Part print with two shaded views. Sizes in mm from the minimum x, y, z corner. Give positions to 0.01 mm unless a question says otherwise; leave off trailing zeros. Order: outer loops, then holes, each group sorted by start corner. A loop starts at its lowest first (then second) coordinate and runs counter-clockwise, first axis right, second up. Notation, with made-up numbers: (40.25, 76.5) -> (60.25, 76.5) arc R23 ccw to (60.25, 113.5) -> close; hole circle Ø9 at (-10, 0). An arc over 180 degrees is marked (long way). Write item = value, one per line. Start each with the question number.
Item 1: Drill centre lines: line 1 along Y through (x, z) = (5.5, 0.4); line 2 along Y through (x, z) = (21, 0.5); line 3 along X through (y, z) = (38, 0.75) (1 decimal). Where is each one in solid material? Low to high.
Item 2: Flat gauge pin, fed straight in: P1, Ø3.5, axis at x = 36.5, y = 36.5, coming from the -Z side. Where does the tip first touch, or does it go through?
Item 3: Band-saw the part on B-B on x = 36.5. Write the cut outline in (y, z).
Item 4: Band-saw the part on C-C on z = 0.8. Write the cut outline in (x, y).
Item 5: Band-saw the part on A-A on y = 21. Write the cut outline in (x, z).
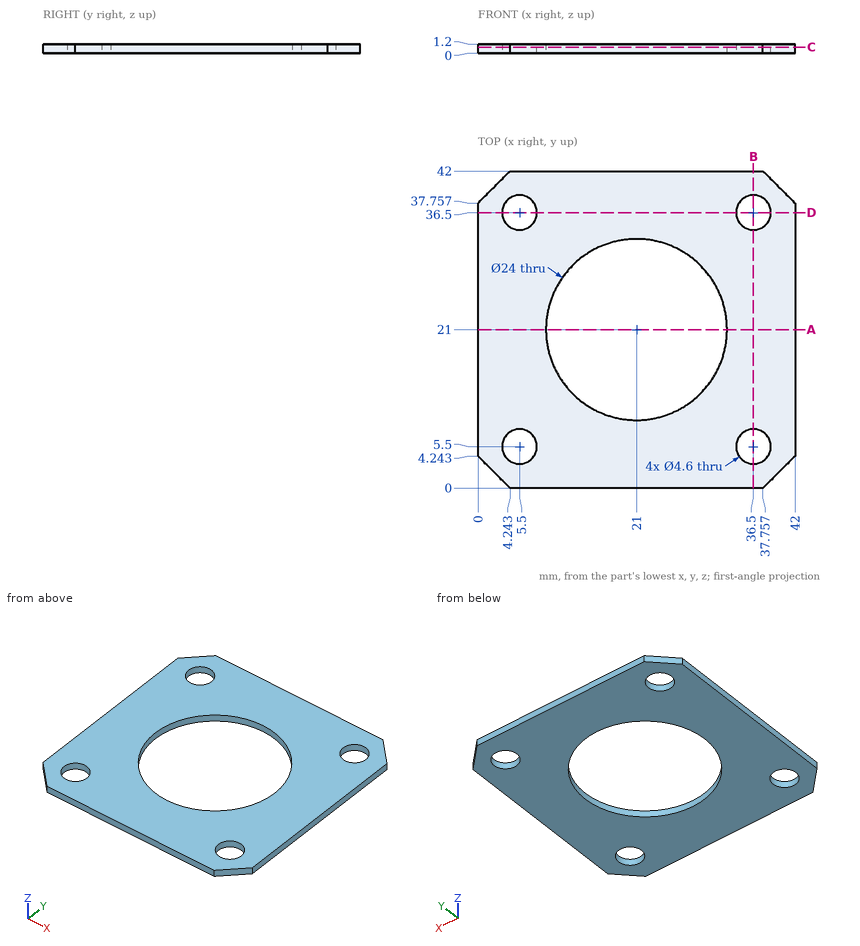
Values found:
q1.line_1 = 0 to 3.2, 7.8 to 34.2, 38.8 to 42
q1.line_2 = 0 to 9, 33 to 42
q1.line_3 = 0.2 to 3.8, 7.2 to 34.8, 38.2 to 41.8
q2.P1 = through
q3.outline = (0, 0) -> (3.2, 0) -> (3.2, 1.2) -> (0, 1.2) -> close; (7.8, 0) -> (34.2, 0) -> (34.2, 1.2) -> (7.8, 1.2) -> close; (38.8, 0) -> (42, 0) -> (42, 1.2) -> (38.8, 1.2) -> close
q4.outline = (0, 4.24) -> (4.24, 0) -> (37.76, 0) -> (42, 4.24) -> (42, 37.76) -> (37.76, 42) -> (4.24, 42) -> (0, 37.76) -> close; hole circle Ø4.6 at (5.5, 5.5); hole circle Ø4.6 at (5.5, 36.5); hole circle Ø24 at (21, 21); hole circle Ø4.6 at (36.5, 5.5); hole circle Ø4.6 at (36.5, 36.5)
q5.outline = (0, 0) -> (9, 0) -> (9, 1.2) -> (0, 1.2) -> close; (33, 0) -> (42, 0) -> (42, 1.2) -> (33, 1.2) -> close
